Autodesk Fusion 360 part; units mm, degrees
sketch "Schizzo1" plane through (0, 0, 0) normal (0, 0, 1) x (1, 0, 0)
  line L0 (0, 0) -> (10, 0)
  line L1 (10, 0) -> (10, 2)
  line L2 (10, 2) -> (0, 2)
  line L3 (0, 2) -> (0, 0)
  line L4 (0, 2) -> (2.5, 2)
  line L5 (2.5, 2) -> (2.5, 4)
  line L6 (2.5, 4) -> (0, 4)
  line L7 (0, 4) -> (0, 2)
  line L8 (0, 4) -> (10, 4)
  line L9 (10, 4) -> (10, 6)
  line L10 (10, 6) -> (0, 6)
  line L11 (0, 6) -> (0, 4)
  dimension "d1" = 10
  dimension "d2" = 2
  dimension "d3" = 2
sketch "Schizzo2" plane through (0, 0, 0) normal (0, 0, 1) x (1, 0, 0)
  line L0 (0, 0) -> (30, 0)
  line L1 (30, 0) -> (30, 3)
  line L2 (30, 3) -> (0, 3)
  line L3 (0, 3) -> (0, 0)
  line L4 (0, 3) -> (10, 3)
  line L5 (10, 3) -> (10, 6)
  line L6 (10, 6) -> (0, 6)
  line L7 (0, 6) -> (0, 3)
  line L8 (0, 6) -> (30, 6)
  line L9 (30, 6) -> (30, 9)
  line L10 (30, 9) -> (0, 9)
  line L11 (0, 9) -> (0, 6)
extrude "Estrusione2" add sketch "Schizzo2" along normal blind 50
fillet "Raccordo3" radius 4.5 2 edges at (0, 0, 25) (0, 9, 25)
fillet "Raccordo4" radius 1.5 4 edges at (30, 0, 25) (30, 3, 25) (30, 6, 25) (30, 9, 25)
extrude "Estrusione3" cut 1 faces at (10, 4, 33.3333) along direction (-1, 0, 0) blind 6
extrude "Estrusione1" [suppressed]
fillet "Raccordo1" [suppressed]
fillet "Raccordo2" [suppressed]
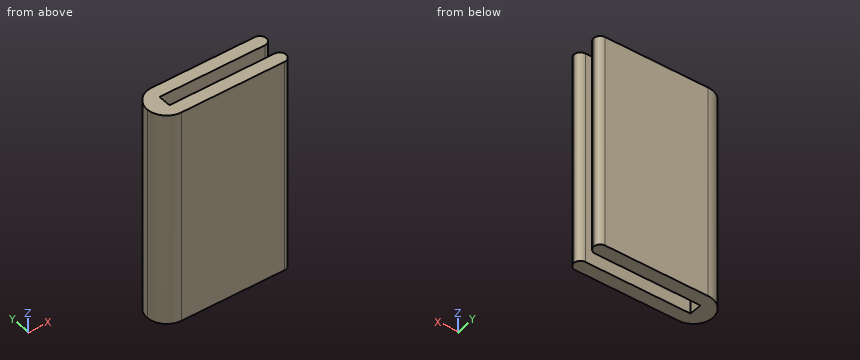
CAD build for the part. Positions are in the model's coordinates, mm. Coordinates: 2 decimals unless noted, no trailing zeros. Order: outer loops, then holes, each group sorted by start corner. A loop starts at its lowest first (then second) coordinate and runs counter-clockwise, first axis right, second up. Notation, with made-up numbers: (-21.5, -18.5) -> (-17.5, -18.5) arc R27 cw to (-17.5, 17.5) -> close; hole circle Ø6 at (33.25, -0.75). An arc over 180 degrees is marked (long way). Use one line per item in the form item = value. Start each with the question number.
1) Band-saw the part on D-D on y = 2. Give the cut face in (x, z).
2) Drop flat-ended pins along their axis: pin 1 (2 mm diameter, centred on y = 7, z = 20.5, fed in from -X); pin 2 (0.9 mm diameter, centred on y = 5, z = 23, fed in from +X). Give the stop position or say it passes through.
3) Band-saw the part on C-C on y = 6.5. Give the cut face in (x, z).
4) Drill centre lines: L1, parallel to Y at x = 25.25, z = 25.5; L2, parallel to X at y = 4.75, z = 41.5; L3, parallel to X at y = 0.75, z = 6.5. Where is each one in solid material? Low to high. Write a range as [from, to].
5) Band-saw the part on A-A on x = 12.75. Give the cut face in (y, z), then the cut area to 3 significant figures.
Entries:
q1.outline = (0.76, 0) -> (29.91, 0) -> (29.91, 50) -> (0.76, 50) -> close
q2.pin_1 = 0.26
q2.pin_2 = 4
q3.outline = (0.47, 0) -> (29.62, 0) -> (29.62, 50) -> (0.47, 50) -> close
q4.L1 = [0, 3], [6, 9]
q4.L2 = [0.01, 4]
q4.L3 = [2.01, 29.8]
q5.outline = (0, 0) -> (3, 0) -> (3, 50) -> (0, 50) -> close; (6, 0) -> (9, 0) -> (9, 50) -> (6, 50) -> close
q5.area = 300 mm2
